Geometry check sheet. Reference: drawing and pictorial views, mm from the part's lowest x, y, z. A direction names the side the tool comes from. Coordinates: 2 decimals unless noted, no trailing zeros. Loops run counter-clockwise (first coordinate to the right, second up) from the corner with the lowest first, then second, coordinate; pieces in that order, holes last. Notation, with made-up numbers: (3.5, 1.25) -> (59.5, 1.25) arc R26 ccw to (59.5, 32.25) -> close; hole circle Ø8 at (54.5, 13.5). An arc over 180 degrees is marked (long way). Use one line per item in the form item = value.
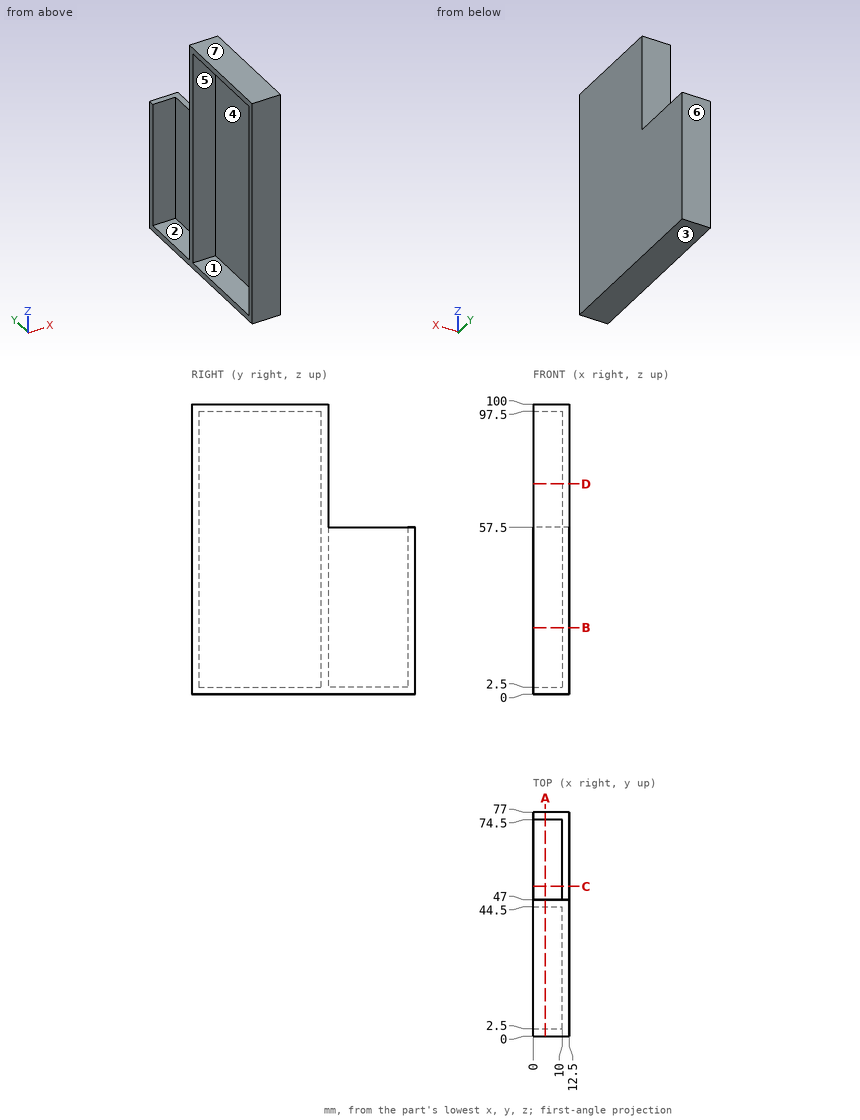
(1) Section check D-D, the plane z = 72.5. Record the boundary of the cut face in (x, y), plus the area to 4 significant figures.
Established:
outline = (0, 0) -> (12.5, 0) -> (12.5, 47) -> (0, 47) -> (0, 44.5) -> (10, 44.5) -> (10, 2.5) -> (0, 2.5) -> close
area = 167.5 mm²
(2) Mould release check, pull along Y, two halves, no side actions. Record for the marked faces 4, 5, 6 and 7: +Y half, -Y half, draft (parallel to the pull), parting line (faces both ways), or undercut.
Established:
face_4 = undercut
face_5 = undercut
face_6 = +Y half
face_7 = draft
(3) Tool access check on the marked faces 1, 2 and 3. Record the directions out of +Z, -Z, +X, -X, +Y, -Y that give a thin tool (end or side, any length) a straight path to the whole face; none if there is none.
Established:
face_1 = -X
face_2 = +Z, -X
face_3 = -Z, +X, -X, +Y, -Y
(4) Section check A-A, the plane x = 4.25. Record the boundary of the cut face in (y, z).
Established:
outline = (0, 0) -> (77, 0) -> (77, 57.5) -> (74.5, 57.5) -> (74.5, 2.5) -> (47, 2.5) -> (47, 100) -> (0, 100) -> close; hole (2.5, 2.5) -> (44.5, 2.5) -> (44.5, 97.5) -> (2.5, 97.5) -> close
(5) Section check C-C, the plane y = 51.5. Record the boundary of the cut face in (x, z).
Established:
outline = (0, 0) -> (12.5, 0) -> (12.5, 57.5) -> (10, 57.5) -> (10, 2.5) -> (0, 2.5) -> close
(6) Go/stop test with flat-tipped pins: P1, Ø1.5, axis at x = 4, z = 65.5, coming from the +Y side; P2, Ø3, axis at x = 7, y = 54.5, coming from the +Z side; P3, Ø6, axis at y = 9, z = 33.5, coming from the -X side. Record where each tip stops, or that it passes through.
Established:
P1 = 47
P2 = 2.5
P3 = 10
(7) Section check B-B, the plane z = 23. Record the boundary of the cut face in (x, y), plus the area to 4 significant figures.
Established:
outline = (0, 0) -> (12.5, 0) -> (12.5, 77) -> (0, 77) -> (0, 74.5) -> (10, 74.5) -> (10, 47) -> (0, 47) -> (0, 44.5) -> (10, 44.5) -> (10, 2.5) -> (0, 2.5) -> close
area = 267.5 mm²
(8) Scan lines: line 1 along Y through (x, z) = (6, 48); line 2 along Z through (x, y) = (4, 28.5); line 3 along Y through (x, z) = (2.75, 82.5). Record each from-to range of solid material in increasing order.
Established:
line_1 = 0 to 2.5, 44.5 to 47, 74.5 to 77
line_2 = 0 to 2.5, 97.5 to 100
line_3 = 0 to 2.5, 44.5 to 47
